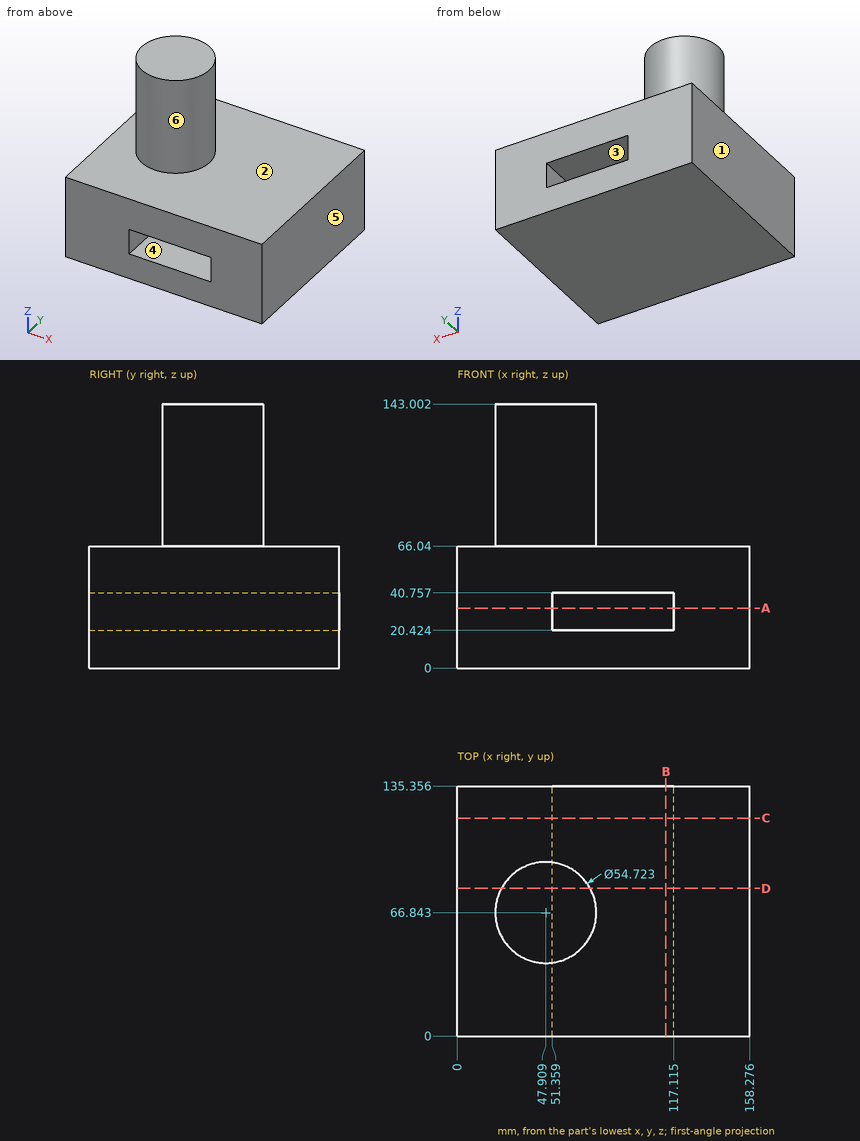
Verification items for this drawing (mm, ordinates from the low corner). A direction names the side the tool comes from. Coordinates: 2 decimals unless noted, no trailing zeros. Loops run counter-clockwise (first coordinate to the right, second up) from the corner with the lowest first, then second, coordinate; pieces in that order, holes last. Notation, with made-up numbers: (-10.5, 67.25) - (13.5, 67.25) arc R7 ccw to (13.5, 77.25) - close; hole circle Ø2 at (-2, 23.5). An arc over 180 degrees is marked (long way). One line per item, written item: value. Start each with the question number.
(1) Cross-section at C-C on y = 118. Enter the section's corners in (x, z) (1 decimal).
(2) Mould release check, pull along X, two halves, no side actions. Record for the marked faces 1, 2, 3 and 4: released by +X, released by -X, zero draft, split by the parting line, or undercut.
(3) Depth check by flat-ended pin: P1, Ø5, axis at y = 49.5, z = 96, coming from the -X side; P2, Ø8, axis at x = 64.5, z = 103.5, coming from the +Y side (1 decimal); P3, Ø8, axis at x = 34, z = 102.5, coming from the -Y side. Enter the tip coordinate at first touch or a pass-through.
(4) Cross-section at A-A on z = 32.5. Enter the section's corners in (x, y) (1 decimal), plus the area to 3 significant figures.
(5) Material ranges on line 1 (Z direction, x = 53, y = 76.5) (1 decimal); line 2 (X direction, y = 120, z = 35) (1 decimal); line 3 (Z direction, x = 111, y = 26) (1 decimal), recorded low to high. Write a range as [from, to].
(6) Cross-section at B-B on x = 113. Enter the section's corners in (y, z) (1 decimal).
(7) Tool access check on the marked faces 5 and 6. Record the directions out of +Z, -Z, +X, -X, +Y, -Y that give a thin tool (end or side, any length) a straight path to the whole face; none if there is none.
(8) Cross-section at D-D on y = 80. Enter the section's corners in (x, z) (1 decimal), plus the area to 3 significant figures.
Results below:
1. outline: (0, 0) - (158.3, 0) - (158.3, 66) - (0, 66) - close; hole (51.4, 20.4) - (117.1, 20.4) - (117.1, 40.8) - (51.4, 40.8) - close
2. face 1: released by -X
2. face 2: zero draft
2. face 3: undercut
2. face 4: undercut
3. P1: stops at x = 24.92
3. P2: stops at y = 91.1
3. P3: stops at y = 41.34
4. outline: (0, 0) - (51.4, 0) - (51.4, 135.4) - (0, 135.4) - close; (117.1, 0) - (158.3, 0) - (158.3, 135.4) - (117.1, 135.4) - close
4. area: 12,500 mm2
5. line 1: z = [0, 20.4], [40.8, 143]
5. line 2: x = [0, 51.4], [117.1, 158.3]
5. line 3: z = [0, 20.4], [40.8, 66]
6. outline: (0, 0) - (135.4, 0) - (135.4, 20.4) - (0, 20.4) - close; (0, 40.8) - (135.4, 40.8) - (135.4, 66) - (0, 66) - close
7. face 5: +Z, -Z, +X, +Y, -Y
7. face 6: +Z
8. outline: (0, 0) - (158.3, 0) - (158.3, 66) - (71.9, 66) - (71.9, 143) - (23.9, 143) - (23.9, 66) - (0, 66) - close; hole (51.4, 20.4) - (117.1, 20.4) - (117.1, 40.8) - (51.4, 40.8) - close
8. area: 12,800 mm2
